Part model, mm, in its own coordinate system. Round coordinates to 2 decimals unless told otherwise and drop trailing zeros. Order: outer loops, then holes, each group sorted by start corner. A loop starts at its lowest first (then second) coordinate and runs counter-clockwise, first axis right, second up. Notation, with made-up numbers: (-5, 26.25) - (2, 26.25) arc R19 cw to (2, 40.25) - close; hole circle Ø5 at (40.25, -0.75). An arc over 180 degrees is marked (long way). Return JSON: item names as keys, results as strings. Group by question number.
Item 1: Drop a flat-ended pin along its axis: pin 1 (5 mm diameter, centred on x = 5.5, y = 1.5, fed in from -Z). Give the stop position or say it passes through.
Item 2: Saw through at A-A on z = 0.6. List the corners of the cut face in (x, y) (1 decimal), and give its area (3 significant figures).
Item 3: Probe probe 1 along X at (y, z) = (15, 1.1); probe 2 along X at (y, z) = (16, 0.25). List the from-to ranges inside material, lowest first.
Autodesk Inventor part; units mm, degrees
ref_plane "YZ Plane" through (0, 0, 0) normal (1, 0, 0) x (0, 1, 0)
ref_plane "XZ Plane" through (0, 0, 0) normal (0, 1, 0) x (-1, 0, 0)
ref_plane "XY Plane" through (0, 0, 0) normal (0, 0, 1) x (1, 0, 0)
sketch "Sketch1" plane through (0, 0, 0) normal (0, 0, 1) x (1, 0, 0)
  line L0 (-241.3, -22.225) -> (241.3, -22.225)
  line L1 (241.3, -22.225) -> (241.3, 22.225)
  line L2 (241.3, 22.225) -> (-241.3, 22.225)
  line L3 (-241.3, 22.225) -> (-241.3, -22.225)
  line L4 (-241.3, -22.225) -> (241.3, 22.225) construction
  line L5 (241.3, -22.225) -> (-241.3, 22.225) construction
  point P0 (0, 0)
  dimension "d0" = 482.6
  dimension "d1" = 44.45
extrude "Extrusion1" add sketch "Sketch1" along normal blind 2
sketch "Sketch2" plane through (0, 0, 2) normal (0, 0, 1) x (1, 0, 0)
  line L0 (-235.2675, 15.875) -> (-228.9175, 15.875) construction
  line L1 (-235.2675, 10.875) -> (-228.9175, 10.875)
  line L2 (-228.9175, 20.875) -> (-235.2675, 20.875)
  arc A0 (-235.2675, 20.875) -> (-235.2675, 10.875) centre (-235.2675, 15.875) ccw
  arc A1 (-228.9175, 10.875) -> (-228.9175, 20.875) centre (-228.9175, 15.875) ccw
  line L3 (241.3, 22.225) -> (-241.3, 22.225)
  line L4 (-241.3, 22.225) -> (-241.3, -22.225)
  line L5 (-241.3, 0) -> (241.3, 0) construction
  line L6 (0, 22.225) -> (0, -22.225) construction
  line L7 (-235.2675, -15.875) -> (-228.9175, -15.875) construction
  line L8 (-235.2675, -10.875) -> (-228.9175, -10.875)
  line L9 (-228.9175, -20.875) -> (-235.2675, -20.875)
  arc A2 (-235.2675, -10.875) -> (-235.2675, -20.875) centre (-235.2675, -15.875) ccw
  arc A3 (-228.9175, -20.875) -> (-228.9175, -10.875) centre (-228.9175, -15.875) ccw
  line L10 (235.2675, 15.875) -> (228.9175, 15.875) construction
  line L11 (235.2675, 10.875) -> (228.9175, 10.875)
  line L12 (228.9175, 20.875) -> (235.2675, 20.875)
  arc A4 (235.2675, 10.875) -> (235.2675, 20.875) centre (235.2675, 15.875) ccw
  arc A5 (228.9175, 20.875) -> (228.9175, 10.875) centre (228.9175, 15.875) ccw
  line L13 (235.2675, -15.875) -> (228.9175, -15.875) construction
  line L14 (235.2675, -10.875) -> (228.9175, -10.875)
  line L15 (228.9175, -20.875) -> (235.2675, -20.875)
  arc A6 (235.2675, -20.875) -> (235.2675, -10.875) centre (235.2675, -15.875) ccw
  arc A7 (228.9175, -10.875) -> (228.9175, -20.875) centre (228.9175, -15.875) ccw
  point P0 (0, 0)
  point P1 (-232.0925, 15.875)
  point P2 (-232.0925, -15.875)
  point P3 (232.0925, 15.875)
  point P4 (232.0925, -15.875)
  dimension "d13" = 5
  dimension "d14" = 6.35
  dimension "d15" = 6.35
  dimension "d16" = 9.2075
extrude "Extrusion2" cut sketch "Sketch2" against normal up to surface (2 mm away)
properties part number "PatchPanel_front"
Filled in:
{
 "1": {"pin 1": "stops at z = 0"},
 "2": {"outline": "(-241.3, -22.2) - (241.3, -22.2) - (241.3, 22.2) - (-241.3, 22.2) - close; hole (-235.3, -20.9) - (-228.9, -20.9) arc R5 ccw to (-228.9, -10.9) - (-235.3, -10.9) arc R5 ccw to start; hole (-235.3, 10.9) - (-228.9, 10.9) arc R5 ccw to (-228.9, 20.9) - (-235.3, 20.9) arc R5 ccw to start; hole (228.9, -20.9) - (235.3, -20.9) arc R5 ccw to (235.3, -10.9) - (228.9, -10.9) arc R5 ccw to start; hole (228.9, 10.9) - (235.3, 10.9) arc R5 ccw to (235.3, 20.9) - (228.9, 20.9) arc R5 ccw to start", "area": "20,900 mm^2"},
 "3": {"probe 1": "x = -241.3 to -240.19, -223.99 to 223.99, 240.19 to 241.3", "probe 2": "x = -241.3 to -240.27, -223.92 to 223.92, 240.27 to 241.3"}
}
